The figure shows three views and two pictorial views of one solid part (mm, origin at its lowest corner). Answer the questions. Coordinates: 2 decimals unless noted, no trailing zeros. Write each loop counter-clockwise with the first axis right and the second up, starting at its lowest first coordinate (ties: lowest second). Pieces come first, ordered by that corner, then holes. Notation, with made-up numbers: (38.5, 33) -> (42.5, 33) arc R11 cw to (42.5, 44) -> close; hole circle Ø6 at (-23, 69). An arc over 180 degrees is marked (long way). Use CSV: the item, a comma, the result in double quotes. Start each with the question number.
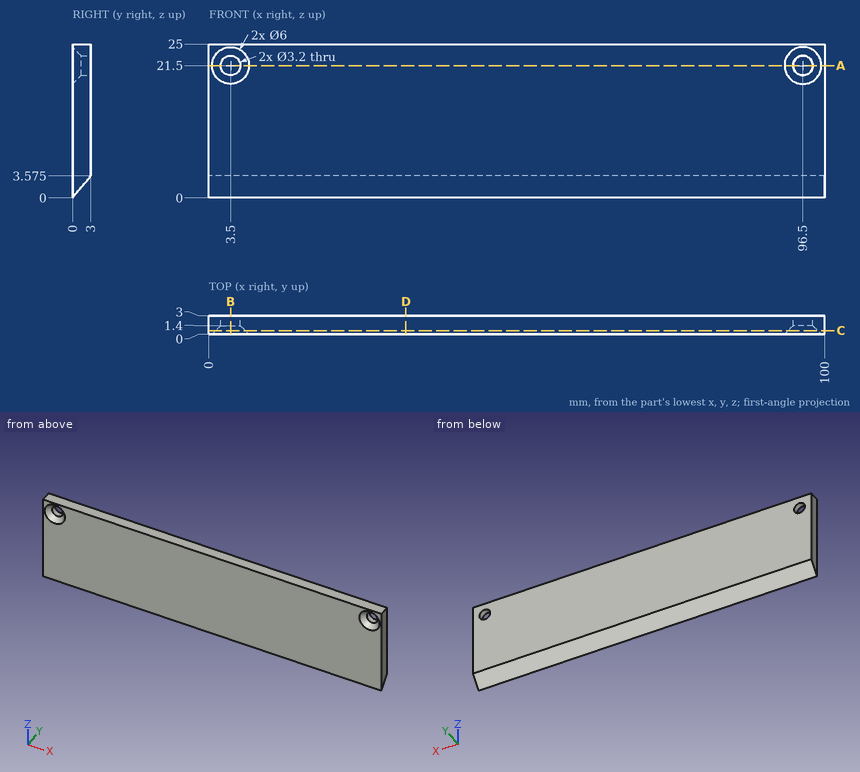
1) Section C-C, the plane y = 0.6 is taken. Give the vertices of the cut face in (x, z) (1 decimal).
2) This flat-tipped pin is pushed along its axis until it touches: pin 1 (2 mm diameter, centred on x = 33.5, z = 12.5, fed in from -Y). Where does it stop, or does it pass through?
3) Section D-D, the plane x = 32 is taken. Give the vertices of the cut face in (y, z) (1 decimal).
4) Section B-B, the plane x = 3.5 is taken. Give the vertices of the cut face in (y, z) (1 decimal).
5) Find the intervals of material crossed by line 1 along X through (y, z) = (2.45, 21.5); line 2 along Z through (x, y) = (3.5, 1.9) (1 decimal); line 3 along Z through (x, y) = (96.5, 2) (1 decimal), in increasing order.
6) Section A-A, the plane z = 21.5 is taken. Give the vertices of the cut face in (x, y).
The answers:
1,outline,"(0, 0.7) -> (100, 0.7) -> (100, 25) -> (0, 25) -> close; hole circle Ø4.8 at (3.5, 21.5); hole circle Ø4.8 at (96.5, 21.5)"
2,pin 1,"stops at y = 0"
3,outline,"(0, 0) -> (3, 3.6) -> (3, 25) -> (0, 25) -> close"
4,outline,"(0, 0) -> (3, 3.6) -> (3, 19.9) -> (1.4, 19.9) -> (0, 18.5) -> close; (0, 24.5) -> (1.4, 23.1) -> (3, 23.1) -> (3, 25) -> (0, 25) -> close"
5,line 1,"x = 0 to 1.9, 5.1 to 94.9, 98.1 to 100"
5,line 2,"z = 2.3 to 19.9, 23.1 to 25"
5,line 3,"z = 2.4 to 19.9, 23.1 to 25"
6,outline,"(0, 0) -> (0.5, 0) -> (1.9, 1.4) -> (1.9, 3) -> (0, 3) -> close; (5.1, 1.4) -> (6.5, 0) -> (93.5, 0) -> (94.9, 1.4) -> (94.9, 3) -> (5.1, 3) -> close; (98.1, 1.4) -> (99.5, 0) -> (100, 0) -> (100, 3) -> (98.1, 3) -> close"
